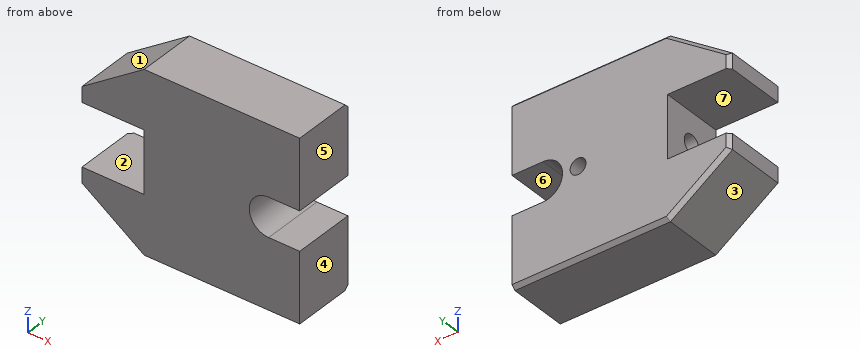
Autodesk Inventor part; units mm, degrees
ref_plane "YZ Plane" through (0, 0, 0) normal (1, 0, 0) x (0, 1, 0)
ref_plane "XZ Plane" through (0, 0, 0) normal (0, 1, 0) x (-1, 0, 0)
ref_plane "XY Plane" through (0, 0, 0) normal (0, 0, 1) x (1, 0, 0)
sketch "Sketch1" plane through (0, 0, 0) normal (0, 1, 0) x (-1, 0, 0)
  line L0 (0, -51.1175) -> (0, 51.1175)
  line L1 (-17.78, 0) -> (106.68, 0)
  line L2 (106.68, 0) -> (-17.78, 0)
  line L3 (0, -51.1175) -> (0, 51.1175)
  line L4 (63.5, 36.5125) -> (0, 36.5125)
  line L5 (0, -36.5125) -> (63.5, -36.5125)
  line L6 (0, 36.5125) -> (63.5, 36.5125)
  line L7 (88.9, 18.9865) -> (63.5, 36.5125)
  line L8 (88.9, 12.6873) -> (63.5, 12.6873)
  line L9 (63.5, 12.6873) -> (63.5, 0)
  line L10 (88.9, -18.9865) -> (63.5, -36.5125)
  line L11 (88.9, -12.6873) -> (63.5, -12.6873)
  line L12 (63.5, -12.6873) -> (63.5, 0)
  line L13 (88.9, 18.9865) -> (88.9, 12.6873)
  line L14 (88.9, -12.6873) -> (88.9, -18.9865)
  line L15 (0, 7.9375) -> (12.6873, 7.9375)
  line L16 (12.6873, -7.9375) -> (0, -7.9375)
  arc A0 (12.6873, -7.9375) -> (12.6873, 7.9375) centre (12.6873, 0) ccw
  line L17 (0, 36.5125) -> (0, 7.9375)
  line L18 (0, -7.9375) -> (0, -36.5125)
  point P0 (0, 0)
  point P1 (0, 0)
  point P2 (0, 36.5125)
  point P3 (0, -7.9375)
  dimension "d1" = 73.025
  dimension "d2" = 63.5
  dimension "d4" = 17.526
  dimension "d5" = 88.9
  dimension "d7" = 23.8252
  dimension "d10" = 12.6873
  dimension "d11" = 15.875
  dimension "d12" = 36.5125
extrude "Extrusion1" add sketch "Sketch1" along normal blind 25.4 contours L0 L16 A0 L1 L12 L11 L14 L10 L5 | L0 L4 L7 L13 L8 L9 L1 A0 L15
chamfer "Chamfer1" distance 1.524 angle 45 6 edges at (-31.75, 25.4, 36.5125) (-76.2, 25.4, 27.7495) (-88.9, 25.4, 15.8369) (-31.75, 25.4, -36.5125) (-76.2, 25.4, -27.7495) (-88.9, 25.4, -15.8369)
sketch "Sketch2" plane through (0, 25.4, 0) normal (0, 1, 0) x (1, 0, 0)
  point P0 (0, 0)
  point P1 (-26.9748, 0)
  dimension "d18" = 26.9748
hole "Hole1" at (-26.9748, 25.4, 0) direction (0, -1, 0) diameter 6.477 depth 14.2748 tip angle 118
sketch "Sketch3" plane through (-63.5, 0, -12.6873) normal (-1, 0, 0) x (0, 0, 1)
  line L0 (0, 0) -> (25.3746, 0)
  point P0 (12.6873, 0)
  point P1 (12.6873, 12.7)
  point P2 (12.6873, 0)
  dimension "d26" = 12.7
hole "Hole2" at (-63.5, 12.7, 0) direction (1, 0, 0) diameter 7.7978 depth 19.05 tip angle 118
properties part number "Ch7(5) Part 1 Base"
The listing builds one solid part. Answer for the finished solid, in the listing's coordinates (mm). Face numbers are marked on the shaded views. A direction names the side the tool comes from. Coordinates: 2 decimals unless noted, no trailing zeros. Loops run counter-clockwise (first coordinate to the right, second up) from the corner with the lowest first, then second, coordinate; pieces in that order, holes last. Notation, with made-up numbers: M 87,43.5 L 100,43.5 A21 ccw 100,82.5 Z; hole C -40,80 d10. An arc over 180 degrees is marked long. Answer as a JSON object with one key per item and string values. Group by question number.
Item 1: Section C-C (y = 4.5) is taken. Write down the section's boundary in (x, z) (1 decimal), and give its area (3 significant figures).
Item 2: Which of the six approach directions +Z, -Z, +X, -X, +Y, -Y give full straight-line access (tool end or side, diameter ignored) to the marked faces 5, 6 and 7?
Item 3: Determine the mould class of the marked faces 1, 2, 3 and 4 for opening direction Z: +Z half, -Z half, draft (parallel to the pull), parting line (faces both ways), or undercut.
Item 4: Section A-A (x = -46.5) is taken. Write down the section's boundary in (y, z), and give its area (3 significant figures).
Item 5: Section D-D (z = -25.5) is taken. Write down the section's boundary in (x, y).
Item 6: Section B-B (x = -67.5) is taken. Write down the section's boundary in (y, z).
Item 7: Each of these flat-tipped pins is pushed along its axis until it touches: P1, Ø7.5, axis at y = 13.5, z = -6, coming from the -X side; P2, Ø8, axis at y = 16, z = -9.5, coming from the -X side; P3, Ø2, axis at y = 17.5, z = 28, coming from the -X side; P4, Ø12, axis at x = -79, y = 3, coming from the +Z side. Where does it stop, or does it pass through?
Item 8: Consider L1, parallel to Z at x = -8, y = 3; L2, parallel to Z at x = -51.5, y = 12.7; L3, parallel to X at y = 21.5, z = 0. Determine where each line is inside the solid, lowest interval first.
Solved:
{
 "1": {"outline": "M -88.9,-19 L -63.5,-36.5 L 0,-36.5 L 0,-7.9 L -12.7,-7.9 A7.9 cw -12.7,7.9 L 0,7.9 L 0,36.5 L -63.5,36.5 L -88.9,19 L -88.9,12.7 L -63.5,12.7 L -63.5,-12.7 L -88.9,-12.7 Z", "area": "5,100 mm2"},
 "2": {"face 5": "+Z, -Z, +X, +Y, -Y", "face 6": "+X, +Y, -Y", "face 7": "-X, +Y, -Y"},
 "3": {"face 1": "+Z half", "face 2": "undercut", "face 3": "-Z half", "face 4": "draft"},
 "4": {"outline": "M 0,-36.51 L 23.88,-36.51 L 25.4,-34.99 L 25.4,34.99 L 23.88,36.51 L 0,36.51 Z; hole C 12.7,0 d7.8", "area": "1,800 mm2"},
 "5": {"outline": "M -79.46,0 L 0,0 L 0,25.4 L -76.78,25.4 L -79.46,23.88 Z"},
 "6": {"outline": "M 0,-33.75 L 23.88,-33.75 L 25.4,-31.9 L 25.4,-12.69 L 0,-12.69 Z; M 0,12.69 L 25.4,12.69 L 25.4,31.9 L 23.88,33.75 L 0,33.75 Z"},
 "7": {"P1": "stops at x = -63.5", "P2": "stops at x = -88.9", "P3": "stops at x = -77.29", "P4": "stops at z = 29.96"},
 "8": {"L1": "z = -36.51 to -7.94, 7.94 to 36.51", "L2": "z = -36.51 to -3.9, 3.9 to 36.51", "L3": "x = -63.5 to -30.21, -23.74 to -20.62"}
}
